from build123d import *

# Parameters (mm, degrees)
SKETCH1_R           = 9.5
BOSS_EXTRUDE1_DEPTH = 10
CUT_EXTRUDE1_START  = -11
SKETCH2_R           = 2.1
CUT_EXTRUDE1_DEPTH  = 12


with BuildPart() as part:
    # Sketch1 → Boss-Extrude1 (new body)
    with BuildSketch(Plane(origin=(0, 0, 0), x_dir=(1, 0, 0), z_dir=(0, 1, 0))):
        Circle(SKETCH1_R)
    extrude(amount=BOSS_EXTRUDE1_DEPTH)

    # Sketch2 → Cut-Extrude1 (cut)
    with BuildSketch(Plane(origin=(0, 10, 0), x_dir=(1, 0, 0), z_dir=(0, 1, 0)).offset(CUT_EXTRUDE1_START)):
        with Locations((5, 0)):
            Circle(SKETCH2_R)
    cut_extrude1 = extrude(amount=CUT_EXTRUDE1_DEPTH, mode=Mode.SUBTRACT)

    # Mirror1: Cut-Extrude1 across plane
    add(cut_extrude1.mirror(Plane(origin=(0, 0, 0), x_dir=(0, 0, 1), z_dir=(1, 0, 0))), mode=Mode.SUBTRACT)


solid = part.part
Geometry: final body of the model. Coordinates: model frame, mm. Round coordinates to 2 decimals unless told otherwise and drop trailing zeros. Order: outer loops, then holes, each group sorted by start corner. A loop starts at its lowest first (then second) coordinate and runs counter-clockwise, first axis right, second up. Notation, with made-up numbers: (8, 7.5) - (65, 7.5) arc R14 cw to (65, 26.5) - close; hole circle Ø11 at (69.5, -10). An arc over 180 degrees is marked (long way). Write each question's results on one line, items separated by ' | '.
Item 1: Section D-D, the plane x = -5. Return the cut outline in (y, z), and give its area (3 significant figures).
Completed:
outline: (0, -8.08) - (10, -8.08) - (10, -2.1) - (0, -2.1) - close; (0, 2.1) - (10, 2.1) - (10, 8.08) - (0, 8.08) - close | area: 120 mm^2
Item 2: Section C-C, the plane z = -4.75. Return the cut outline in (x, y).
Completed:
outline: (-8.23, 0) - (8.23, 0) - (8.23, 10) - (-8.23, 10) - close
Item 3: Material intervals for line 1 along X through (y, z) = (6.75, 0.25); line 2 along X through (y, z) = (2.25, -0.5); line 3 along Z through (x, y) = (-5, 4.75), sorted ascending. Write a range as [from, to].
Completed:
line 1: [-9.5, -7.09], [-2.91, 2.91], [7.09, 9.5] | line 2: [-9.49, -7.04], [-2.96, 2.96], [7.04, 9.49] | line 3: [-8.08, -2.1], [2.1, 8.08]
Item 4: Section B-B, the plane y = 7.25. Return the cut outline in (x, z).
Completed:
outline: circle Ø19 at (0, 0); hole circle Ø4.2 at (-5, 0); hole circle Ø4.2 at (5, 0)
Item 5: Section A-A, the plane x = 4.5. Return the cut outline in (y, z), and give its area (3 significant figures).
Completed:
outline: (0, -8.37) - (10, -8.37) - (10, -2.04) - (0, -2.04) - close; (0, 2.04) - (10, 2.04) - (10, 8.37) - (0, 8.37) - close | area: 127 mm^2
Item 6: First-contact query: pin 1 Ø6 at (x, y) = (-4.5, 6.5) entering from +Z; pin 2 Ø3 at (y, z) = (7, -3.5) entering from -X. Flat tips, straight axial feed; report the tip coordinate or a pass-through.
Completed:
pin 1: z = 9.38 | pin 2: x = -9.29
Item 7: Mould query, pull axis Z, two halves, no side actions, for faces 1 (the cylindrical face through (4.38, 4.93, 8.43)), 2 (the flat face through (0, 10, 0)), 3 (the cylindrical face through (7.003, 4.93, -0.631)). Classes: pulls with the +Z half, pulls with the -Z half, needs draft (parallel to the pull), parting line crosses it, or undercut.
Completed:
face 1: parting line crosses it | face 2: needs draft | face 3: undercut
